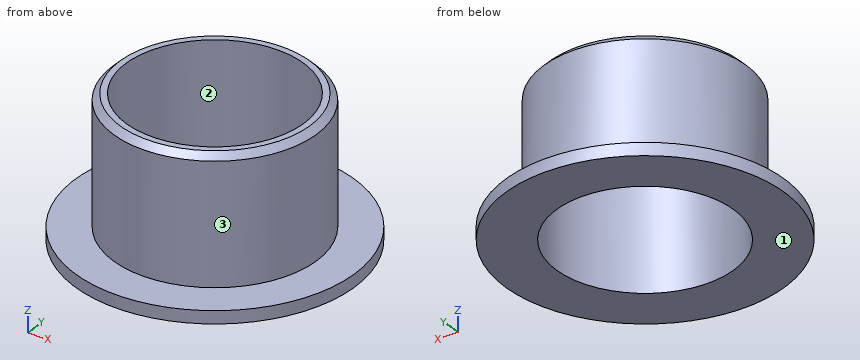
Autodesk Inventor part; units mm, degrees
ref_plane "YZ Plane" through (0, 0, 0) normal (1, 0, 0) x (0, 1, 0)
ref_plane "XZ Plane" through (0, 0, 0) normal (0, 1, 0) x (-1, 0, 0)
ref_plane "XY Plane" through (0, 0, 0) normal (0, 0, 1) x (1, 0, 0)
sketch "スケッチ1" plane through (0, 0, 0) normal (0, 0, 1) x (1, 0, 0)
  circle A0 centre (0, 0) radius 7
  circle A1 centre (0, 0) radius 11
  dimension "d0" = 14
  dimension "d1" = 22
extrude "押し出し1" add sketch "スケッチ1" along normal blind 1
sketch "スケッチ2" plane through (0, 0, 1) normal (0, 0, 1) x (1, 0, 0)
  circle A0 centre (0, 0) radius 8
  circle A1 centre (0, 0) radius 11
  circle A2 centre (0, 0) radius 7
  dimension "d4" = 16
extrude "押し出し2" add sketch "スケッチ2" along normal blind 10 contours A0
chamfer "面取り1" distance 0.5 angle 45 1 edges at (-8, 0, 11)
properties part number "オイレスw5f10-12a" material "アセタール樹脂、黒"
For this review, take the finished solid that the model builds, in its own axes (mm). Face numbers are marked on the shaded views. Coordinates: 2 decimals unless noted, no trailing zeros. Order: outer loops, then holes, each group sorted by start corner. A loop starts at its lowest first (then second) coordinate and runs counter-clockwise, first axis right, second up. Notation, with made-up numbers: (-12.5, 61) -> (-4.5, 61) arc R24 cw to (-4.5, 98) -> close; hole circle Ø11 at (22, 84.25). An arc over 180 degrees is marked (long way). Return JSON: item names as keys, results as strings.
1. We need section A-A on y = 0. Write out the cut boundary in (x, z), and give its area (4 significant figures).
Answer block:
{"outline": "(-11, 0) -> (-7, 0) -> (-7, 11) -> (-7.5, 11) -> (-8, 10.5) -> (-8, 1) -> (-11, 1) -> close; (7, 0) -> (11, 0) -> (11, 1) -> (8, 1) -> (8, 10.5) -> (7.5, 11) -> (7, 11) -> close", "area": "27.75 mm²"}
2. We need section C-C on z = 3.5. Write out the cut boundary in (x, y).
Answer block:
{"outline": "circle Ø16 at (0, 0); hole circle Ø14 at (0, 0)"}
3. We need section D-D on y = 9. Write out the cut boundary in (x, z), and give its area (3 significant figures).
Answer block:
{"outline": "(-6.32, 0) -> (6.32, 0) -> (6.32, 1) -> (-6.32, 1) -> close", "area": "12.6 mm²"}
4. For line 1 (Y direction, x = 0, z = 2.5); line 2 (X direction, y = -4.25, z = 8.25), list the stretches that pass through material, from the lowest coordinate up. Write a range as from..to.
Answer block:
{"line 1": "-8..-7, 7..8", "line 2": "-6.78..-5.56, 5.56..6.78"}
5. For pin 1 Ø2 at (y, z) = (-6, 2.5) entering from +X (3 decimals); pin 2 Ø5 at (y, z) = (0.5, 8.5) entering from -X; pin 3 Ø1.5 at (y, z) = (0, 6) entering from +X; pin 4 Ø11 at (x, y) = (-0.5, 2.5) entering from +Z, all flat-tipped, find the tip position at first contact; note any pin that passes through.
Answer block:
{"pin 1": "x = 6.245", "pin 2": "x = -8", "pin 3": "x = 8", "pin 4": "z = 11"}
6. The part is to be moulded in two halves that separate along X. For the marked faces 1, 2 and 3, say which applies: +X half, -X half, draft (parallel to the pull), parting line (faces both ways), or undercut.
Answer block:
{"face 1": "draft", "face 2": "undercut", "face 3": "parting line"}
